The listing builds one solid part. Answer for the finished solid, in the listing's coordinates (mm). Give positions to 0.01 mm unless a question says otherwise; leave off trailing zeros. Order: outer loops, then holes, each group sorted by start corner. A loop starts at its lowest first (then second) coordinate and runs counter-clockwise, first axis right, second up. Notation, with made-up numbers: (-4, 7) - (51, 7) arc R22 ccw to (51, 20) - close; hole circle Ø3 at (19.25, 66.5). An arc over 180 degrees is marked (long way). Answer in a Markdown table with one row per item.
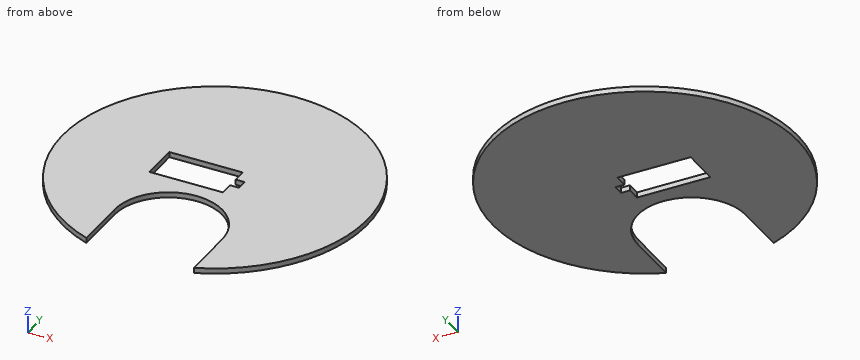
from build123d import *

# Parameters (mm, degrees)
ESQUISSE1_R              = 85
BOSS_EXTRU_1_DEPTH       = 3
ESQUISSE2_R              = 1
ENL_V_MAT_EXTRU_1_DEPTH  = 3
ENL_V_MAT_EXTRU_10_DEPTH = 3


with BuildPart() as part:
    # Esquisse1 → Boss.-Extru.1 (new body)
    with BuildSketch(Plane.XY):
        with Locations((-11.197924537, 8.24446622)):
            Circle(ESQUISSE1_R)
    extrude(amount=BOSS_EXTRU_1_DEPTH)

    # Esquisse2 → Enlèv. mat.-Extru.1 (cut)
    # profile 1 of 2: a face of its own
    with BuildSketch(Plane(origin=(0, 0, 0), x_dir=(-1, 0, 0), z_dir=(0, 0, -1))):
        Polygon((-3.802075463, 11.24446622), (-3.802075463, 5.24446622), (1.197924537, 5.24446622), (1.197924537, -2.25553378), (42.197924537, -2.25553378), (42.197924537, 18.74446622), (1.197924537, 18.74446622), (1.197924537, 11.24446622), align=None)
        with Locations((11.197924537, 8.24446622)):
            Circle(ESQUISSE2_R, mode=Mode.SUBTRACT)
    # profile 2 of 2: a face of its own
    with BuildSketch(Plane(origin=(0, 0, 0), x_dir=(-1, 0, 0), z_dir=(0, 0, -1))):
        with Locations((11.197924537, 8.24446622)):
            Circle(ESQUISSE2_R)
    extrude(amount=-ENL_V_MAT_EXTRU_1_DEPTH, mode=Mode.SUBTRACT)

    # Esquisse3 → Enlèv. mat.-Extru.10 (cut)
    with BuildSketch(Plane(origin=(0, 0, 0), x_dir=(-1, 0, 0), z_dir=(0, 0, -1))):
        with BuildLine():
            Line((-18.802075463, -71.285402383), (-18.802075463, -41.285402383))
            ThreePointArc((-18.802075463, -41.285402383), (11.197924537, -11.285402383), (41.197924537, -41.285402383))
            Line((41.197924537, -41.285402383), (41.197924537, -71.285402383))
            ThreePointArc((41.197924537, -71.285402383), (11.197924537, -76.75553378), (-18.802075463, -71.285402383))
        make_face()
    extrude(amount=-ENL_V_MAT_EXTRU_10_DEPTH, mode=Mode.SUBTRACT)


solid = part.part
Item 1: Find section C-C on y = -15. Write down the section's boundary in (x, z), then the cut area to 3 significant figures.
Answer block:
| item | result |
|---|---|
| outline | (-92.96, 0) - (-25.66, 0) - (-25.66, 3) - (-92.96, 3) - close; (3.26, 0) - (70.56, 0) - (70.56, 3) - (3.26, 3) - close |
| area | 404 mm² |
Item 2: Each of these flat-tipped pins is pushed along its axis until it touches: P1, Ø1, axis at y = 39.5, z = 1.5, coming from the -X side; P2, Ø0.9, axis at y = 0.5, z = 2, coming from the -X side; P3, Ø0.9, axis at y = 14.5, z = 2, coming from the -X side. Where does it stop, or does it pass through?
Answer block:
| item | result |
|---|---|
| P1 | x = -90.44 |
| P2 | x = -95.88 |
| P3 | x = -96 |
Item 3: Find section A-A on z = 2.05. Write down the section's boundary in (x, y).
Answer block:
| item | result |
|---|---|
| outline | (-41.2, -71.29) - (-41.2, -41.29) arc R30 cw to (18.8, -41.29) - (18.8, -71.29) arc R85 ccw (long way) to start; hole (-42.2, -2.26) - (-1.2, -2.26) - (-1.2, 5.24) - (3.8, 5.24) - (3.8, 11.24) - (-1.2, 11.24) - (-1.2, 18.74) - (-42.2, 18.74) - close |
Item 4: Find section B-B on x = -4. Write down the section's boundary in (y, z).
Answer block:
| item | result |
|---|---|
| outline | (-12.16, 0) - (-2.26, 0) - (-2.26, 3) - (-12.16, 3) - close; (18.74, 0) - (92.94, 0) - (92.94, 3) - (18.74, 3) - close |
Item 5: Consider line 1 (X direction, y = 7, z = 1.1); line 2 (Y direction, x = -26, z = 1.1); line 3 (Y direction, x = -22.5, z = 1.8). Determine where each line is inside the solid, lowest interval first.
Answer block:
| item | result |
|---|---|
| line 1 | -96.19 to -42.2, 3.8 to 73.79 |
| line 2 | -15.19 to -2.26, 18.74 to 91.95 |
| line 3 | -13.5 to -2.26, 18.74 to 92.49 |
Item 6: Find section D-D on y = 82. Write down the section's boundary in (x, z), then the cut area to 3 significant figures.
Answer block:
| item | result |
|---|---|
| outline | (-53.45, 0) - (31.05, 0) - (31.05, 3) - (-53.45, 3) - close |
| area | 254 mm² |
